Source: CAD feature listing. Evaluate the final solid. Frame: model axes, mm. Face numbers are marked on the shaded views. A direction names the side the tool comes from. Round coordinates to 2 decimals unless told otherwise and drop trailing zeros. Loops run counter-clockwise (first coordinate to the right, second up) from the corner with the lowest first, then second, coordinate; pieces in that order, holes last. Notation, with made-up numbers: M -1.75,4 L 50.25,4 A25 ccw 50.25,31 Z; hole C -7.5,62 d7. An arc over 180 degrees is marked long. One line per item, written item: value.
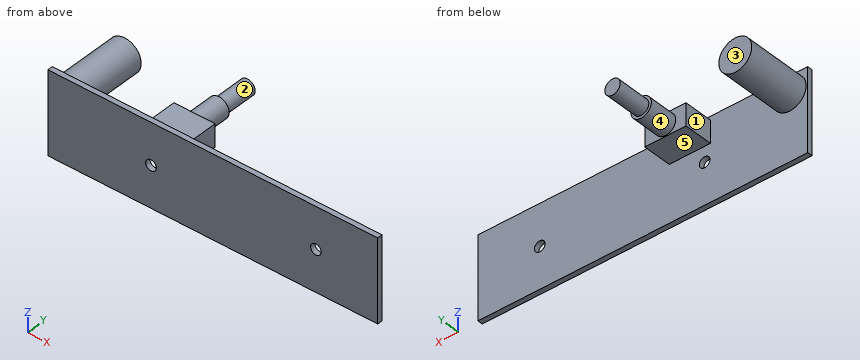
from build123d import *

# Parameters (mm, degrees)
SKETCH1_W                 = 101.6
SKETCH1_H                 = 25.4
BOSS_EXTRUDE1_DEPTH       = 1.5875
F_4_CLEARANCE_HOLE2_D     = 3.2639
F_4_CLEARANCE_HOLE2_DEPTH = 1.5875
SKETCH5_R                 = 5.08
BOSS_EXTRUDE2_DEPTH       = 19.812
SKETCH6_W                 = 12.7
SKETCH6_H                 = 6.858
BOSS_EXTRUDE3_DEPTH       = 8.89
SKETCH7_R                 = 3.175
BOSS_EXTRUDE4_DEPTH       = 8.89
SKETCH8_R                 = 2.38125
BOSS_EXTRUDE5_DEPTH       = 10.414


with BuildPart() as part:
    # Sketch1 → Boss-Extrude1 (new body)
    with BuildSketch(Plane(origin=(0, 0, 0), x_dir=(1, 0, 0), z_dir=(0, 1, 0))):
        with Locations((50.8, 12.7)):
            Rectangle(SKETCH1_W, SKETCH1_H)
    extrude(amount=BOSS_EXTRUDE1_DEPTH)

    # #4 Clearance Hole2
    with Locations(Plane(origin=(0, 1.5875, 0), x_dir=(1, 0, 0), z_dir=(0, 1, 0))):
        with Locations((31.75, 12.7), (82.55, 12.7)):
            Hole(F_4_CLEARANCE_HOLE2_D / 2, depth=F_4_CLEARANCE_HOLE2_DEPTH)

    # Sketch5 → Boss-Extrude2 (add)
    with BuildSketch(Plane(origin=(0, 1.5875, 0), x_dir=(1, 0, 0), z_dir=(0, 1, 0))):
        with Locations((5.588, 5.334)):
            Circle(SKETCH5_R)
    extrude(amount=BOSS_EXTRUDE2_DEPTH)

    # Sketch6 → Boss-Extrude3 (add)
    with BuildSketch(Plane(origin=(0, 1.5875, 0), x_dir=(1, 0, 0), z_dir=(0, 1, 0))):
        with Locations((36.322, 4.572)):
            Rectangle(SKETCH6_W, SKETCH6_H)
    extrude(amount=BOSS_EXTRUDE3_DEPTH)

    # Sketch7 → Boss-Extrude4 (add)
    with BuildSketch(Plane(origin=(0, 10.4775, 0), x_dir=(1, 0, 0), z_dir=(0, 1, 0))):
        with Locations((36.322, 4.572)):
            Circle(SKETCH7_R)
    extrude(amount=BOSS_EXTRUDE4_DEPTH)

    # Sketch8 → Boss-Extrude5 (add)
    with BuildSketch(Plane(origin=(0, 19.3675, 0), x_dir=(1, 0, 0), z_dir=(0, 1, 0))):
        with Locations((36.322, 4.572)):
            Circle(SKETCH8_R)
    extrude(amount=BOSS_EXTRUDE5_DEPTH)


solid = part.part
1. Section query B-B (x = 31.75). Return the cut outline in (y, z).
Report:
outline: M 0,-25.4 L 1.59,-25.4 L 1.59,-14.33 L 0,-14.33 Z; M 0,-11.07 L 1.59,-11.07 L 1.59,-8 L 10.48,-8 L 10.48,-1.14 L 1.59,-1.14 L 1.59,0 L 0,0 Z
2. Section query C-C (x = 82.55). Return the cut outline in (y, z), and give its area (3 significant figures).
Report:
outline: M 0,-25.4 L 1.59,-25.4 L 1.59,-14.33 L 0,-14.33 Z; M 0,-11.07 L 1.59,-11.07 L 1.59,0 L 0,0 Z
area: 35.1 mm2
3. Pin query (flat end, axial travel): pin 1 (5.5 mm diameter, centred on y = 5.5, z = -3.5, fed in from +X); pin 2 (2.5 mm diameter, centred on x = 82.55, z = -12.7, fed in from +Y); pin 3 (2 mm diameter, centred on y = 6, z = -5.5, fed in from -X); pin 4 (1 mm diameter, centred on y = 21.5, z = -7.5, fed in from -X). Return the tip coordinate at first contact, or that it passes through.
Report:
pin 1: stops at x = 42.67
pin 2: passes through
pin 3: stops at x = 0.51
pin 4: stops at x = 0.79
4. Reachability of the marked faces 1, 2 and 3 from +Z, -Z, +X, -X, +Y, -Y: full face, straight path, thin tool, end or side. Return the list, or none.
Report:
face 1: +Z, -Z, +Y
face 2: +Y
face 3: +Z, -Z, -X, +Y
5. Ray query, line 1 (X direction, y = 0.75, z = -12.7); line 2 (X direction, y = 7.75, z = -5.25); line 3 (Y direction, x = 58.5, z = -2). Return the intervals inside material, ascending. Write a range as [from, to].
Report:
line 1: x = [0, 30.12], [33.38, 80.92], [84.18, 101.6]
line 2: x = [0.51, 10.67], [29.97, 42.67]
line 3: y = [0, 1.59]
6. Pull-direction query (X, two-part tool) for the marked faces 4 and 5; classes: released by +X, released by -X, zero draft, split by the parting line, or undercut.
Report:
face 4: undercut
face 5: zero draft
7. Section query A-A (z = -12.7). Return the cut outline in (x, y), and give its area (3 significant figures).
Report:
outline: M 0,0 L 30.12,0 L 30.12,1.59 L 0,1.59 Z; M 33.38,0 L 80.92,0 L 80.92,1.59 L 33.38,1.59 Z; M 84.18,0 L 101.6,0 L 101.6,1.59 L 84.18,1.59 Z
area: 151 mm2
8. Section query D-D (y = 6). Return the cut outline in (x, z), and give its area (3 significant figures).
Report:
outline: C 5.59,-5.33 d10.16; M 29.97,-8 L 42.67,-8 L 42.67,-1.14 L 29.97,-1.14 Z
area: 168 mm2
